Source: CAD feature listing. Evaluate the final solid. Frame: model axes, mm. Face numbers are marked on the shaded views. A direction names the side the tool comes from. Give positions to 0.01 mm unless a question says otherwise; leave off trailing zeros. Order: outer loops, then holes, each group sorted by start corner. A loop starts at its lowest first (then second) coordinate and runs counter-clockwise, first axis right, second up. Notation, with made-up numbers: (11.25, -3) - (52.25, -3) arc R34 cw to (52.25, 36) - close; hole circle Ø5 at (32.5, 47.25). An arc over 180 degrees is marked (long way). Write each question's results on one line, items separated by ' | '. Start each with the question number.
Item 1: Set-up query: the marked faces 1 and 2. Return all of +Z, -Z, +X, -X, +Y, -Y with unobstructed straight access to the full face (end or side cutting, diameter ignored); none if empty.
Item 2: Section B-B on x = 0. Output: boundary loops of the cut face in (y, z) (3 decimals).
Item 3: Section A-A on z = 0. Output: boundary loops of the cut face in (x, y) (3 decimals).
Item 4: Section C-C on y = 12. Output: boundary loops of the cut face in (x, z), and give its area (3 significant figures).
Item 5: Section D-D on z = 7. Output: boundary loops of the cut face in (x, y).
Item 6: Line query: line 1 along Y through (x, z) = (8.75, -2); line 2 along Z through (x, y) = (-0.5, 23.5); line 3 along Z through (x, y) = (-6, 20). Output: solid intervals per line, ascending.
Item 7: Contact query for a flat-ended pin moving along its axis: pin 1 Ø1 at (y, z) = (32, -7.5) entering from +X. Output: stop coordinate, or through.
Autodesk Inventor part; units mm, degrees
ref_plane "YZ Plane" through (0, 0, 0) normal (1, 0, 0) x (0, 1, 0)
ref_plane "XZ Plane" through (0, 0, 0) normal (0, 1, 0) x (-1, 0, 0)
ref_plane "XY Plane" through (0, 0, 0) normal (0, 0, 1) x (1, 0, 0)
sketch "Sketch1" plane through (0, 0, 0) normal (0, 1, 0) x (-1, 0, 0)
  point P0 (0, 0)
sketch "Sketch2" plane through (0, 0, 0) normal (0, 1, 0) x (-1, 0, 0)
  arc A0 (9.1, 7.6681) -> (-9.1, 7.6681) centre (0, 0) ccw
  line L0 (0, 0) -> (9.1, 0)
  line L1 (9.1, 0) -> (-9.1, 0)
  line L2 (-9.1, 0) -> (-9.1, -7.6681)
  line L3 (-9.1, 0) -> (-9.1, 7.6681)
  line L4 (9.1, 0) -> (9.1, -7.6681)
  line L5 (9.1, 0) -> (9.1, 7.6681)
  arc A1 (-9.1, -7.6681) -> (9.1, -7.6681) centre (0, 0) ccw
  dimension "d0" = 23.8
  dimension "d1" = 9.1
  dimension "d2" = 18.2
extrude "Extrusion1" add sketch "Sketch2" along normal blind 30.6
sketch "Sketch3" plane through (0, 30.6, 0) normal (0, 1, 0) x (1, 0, 0)
  circle A0 centre (0, 0) radius 3.075
  dimension "d5" = 6.15
extrude "Extrusion2" add sketch "Sketch3" along normal blind 1.6
sketch "Sketch4" plane through (0, 32.2, 0) normal (0, 1, 0) x (1, 0, 0)
  circle A0 centre (0, 0) radius 1
  dimension "d8" = 2
extrude "Extrusion3" add sketch "Sketch4" along normal blind 15
sketch "Sketch5" plane through (0, 30.6, 0) normal (0, 1, 0) x (1, 0, 0)
  arc A0 (-9.1, -7.6681) -> (9.1, -7.6681) centre (0, 0) ccw
  line L0 (9.1, -7.6681) -> (-9.1, -7.6681)
  circle A1 centre (0, 0) radius 1
  line L1 (0, 0) -> (0, -7.6681)
properties part number "Dc-Motor"
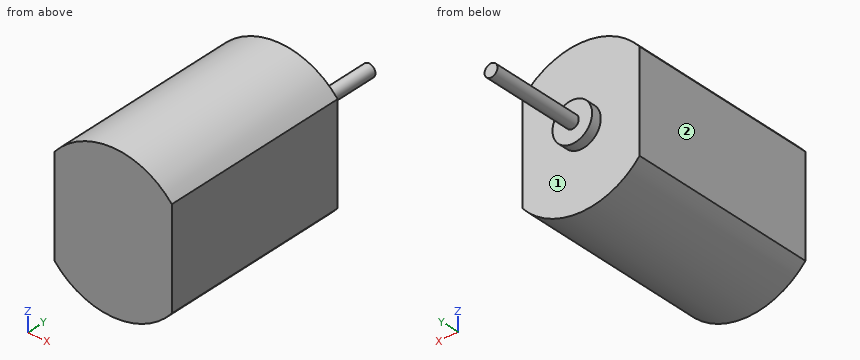
Evaluation:
1) face 1: +Y | face 2: +Z, -Z, -X, +Y, -Y
2) outline: (0, -11.9) - (30.6, -11.9) - (30.6, -3.075) - (32.2, -3.075) - (32.2, -1) - (47.2, -1) - (47.2, 1) - (32.2, 1) - (32.2, 3.075) - (30.6, 3.075) - (30.6, 11.9) - (0, 11.9) - close
3) outline: (-9.1, 0) - (9.1, 0) - (9.1, 30.6) - (3.075, 30.6) - (3.075, 32.2) - (1, 32.2) - (1, 47.2) - (-1, 47.2) - (-1, 32.2) - (-3.075, 32.2) - (-3.075, 30.6) - (-9.1, 30.6) - close
4) outline: (-9.1, -7.67) arc R11.9 ccw to (9.1, -7.67) - (9.1, 7.67) arc R11.9 ccw to (-9.1, 7.67) - close | area: 386 mm^2
5) outline: (-9.1, 0) - (9.1, 0) - (9.1, 30.6) - (-9.1, 30.6) - close
6) line 1: y = 0 to 30.6 | line 2: z = -11.89 to 11.89 | line 3: z = -10.28 to 10.28
7) pin 1: passes through
